The listing builds one solid part. Answer for the finished solid, in the listing's coordinates (mm). A direction names the side the tool comes from. Give positions to 0.01 mm unless a question says otherwise; leave off trailing zeros. Loops run counter-clockwise (first coordinate to the right, second up) from the corner with the lowest first, then second, coordinate; pieces in that order, holes last. Notation, with made-up numbers: M -6,40.25 L 3,40.25 A36 cw 3,77.25 Z; hole C 3,64.25 d5. An arc over 180 degrees is marked long. Return JSON: item names as keys, results as strings.
Autodesk Inventor part; units mm, degrees
ref_plane "YZ Plane" through (0, 0, 0) normal (1, 0, 0) x (0, 1, 0)
ref_plane "XZ Plane" through (0, 0, 0) normal (0, 1, 0) x (-1, 0, 0)
ref_plane "XY Plane" through (0, 0, 0) normal (0, 0, 1) x (1, 0, 0)
sketch "Boceto1" plane through (0, 0, 0) normal (0, 0, 1) x (-1, 0, 0)
  line L0 (-18.5763, -36.3749) -> (-15.5263, -36.3749)
  line L1 (-15.5263, -36.3749) -> (-15.5263, -48.4733)
  line L2 (-15.5263, -48.4733) -> (-5.0037, -48.4733)
  line L3 (-5.0037, -48.4733) -> (-5.0037, -45.4233)
  line L4 (-5.0037, -45.4233) -> (7.1965, -45.4233)
  line L5 (7.1965, -45.4233) -> (7.1965, -48.4733)
  line L6 (7.1965, -48.4733) -> (9.5287, -48.4733)
  line L7 (9.5287, -48.4733) -> (16.194, -48.4733)
  line L8 (16.194, -48.4733) -> (16.194, -47.9303)
  line L9 (16.194, -47.9303) -> (16.194, -45.4233)
  line L10 (16.194, -45.4233) -> (16.194, -36.3411)
  line L11 (16.194, -36.3411) -> (19.2441, -36.3411)
  line L12 (19.2441, -36.3411) -> (19.2441, -24.1748)
  line L13 (19.2444, -24.1748) -> (16.1963, -24.1748)
  line L14 (16.1963, -24.1748) -> (16.1954, -10.116)
  line L15 (16.1954, -10.116) -> (16.194, -6.0779)
  line L16 (16.1918, -6.1454) -> (16.194, -6.0779)
  line L17 (16.194, -6.0779) -> (19.2441, -6.0779)
  line L18 (19.2441, -6.0779) -> (19.2441, 6.1222)
  line L19 (19.2441, 6.1222) -> (16.194, 6.1222)
  line L20 (16.194, 6.1222) -> (16.194, 24.2191)
  line L21 (16.194, 24.2191) -> (19.2441, 24.2191)
  line L22 (19.2441, 24.2191) -> (19.2441, 36.4192)
  line L23 (19.2441, 36.4192) -> (16.194, 36.4192)
  line L24 (16.194, 36.4192) -> (16.194, 45.4676)
  line L25 (16.194, 45.4676) -> (16.194, 48.5176)
  line L26 (16.194, 48.5176) -> (7.1965, 48.5176)
  line L27 (7.1965, 48.5176) -> (7.1965, 45.4676)
  line L28 (7.1965, 45.4676) -> (-3.3262, 45.4676)
  line L29 (-3.3262, 45.4676) -> (-5.0037, 45.4676)
  line L30 (-5.0037, 45.4676) -> (-5.0037, 48.5176)
  line L31 (-5.0037, 48.5176) -> (-15.5263, 48.5176)
  line L32 (-15.5263, 48.5176) -> (-15.5263, 36.4192)
  line L33 (-15.5263, 36.4192) -> (-18.5763, 36.4192)
  line L34 (-18.5763, 36.4192) -> (-18.5763, 24.2191)
  line L35 (-18.5763, 24.2191) -> (-15.5263, 24.2191)
  line L36 (-15.5263, 24.2191) -> (-15.5263, 6.1222)
  line L37 (-15.5263, 6.1222) -> (-18.5763, 6.1222)
  line L38 (-18.5763, 6.1222) -> (-18.5763, -6.0779)
  line L39 (-18.5763, -6.0779) -> (-15.5263, -6.0779)
  line L40 (-15.5263, -6.0779) -> (-15.5263, -24.1748)
  line L41 (-15.5263, -24.1748) -> (-17.5596, -24.1748)
  line L42 (-17.5596, -24.1748) -> (-18.5763, -24.1748)
  line L43 (-18.5763, -24.1748) -> (-18.5763, -36.3749)
  line L44 (-16.0528, -24.1739) -> (-19.1028, -24.1739)
  line L45 (6.6699, 45.4684) -> (4.9416, 45.4684)
  line L46 (-3.8527, -18.4805) -> (-3.8527, -26.614)
  line L47 (-3.8527, -26.614) -> (-6.9027, -26.614)
  line L48 (-6.9027, -26.614) -> (-6.9027, -18.4805)
  line L49 (-6.9027, -18.4805) -> (-3.8527, -18.4805)
  circle A0 centre (1.129, 6.6314) radius 1.0167
  circle A1 centre (4.8907, 0.023) radius 4.575
  circle A2 centre (12.5158, 0.023) radius 1.0167
  circle A3 centre (1.129, -6.5854) radius 1.0167
  point P0 (0, 0)
  dimension "d2" = 96.991
  dimension "d3" = 37.82
extrude "Extrusión1" add sketch "Boceto1" along normal blind 3
properties part number "costat3"
(1) Given pin 1 (1.5 mm diameter, centred on y = 19.5, z = 1.5, fed in from -X); pin 2 (2.5 mm diameter, centred on x = -1.13, y = 6.59, fed in from -Z); pin 3 (0.9 mm diameter, centred on x = -17, z = 1, fed in from +Y), each flat-ended and moving along its own axis, determine where each tip first touches the part or whether it passes through.
Values follow:
{"pin 1": "x = -16.2", "pin 2": "z = 0", "pin 3": "y = 36.34"}
(2) The part is cut by section C-C (z = 1.1). Give the number of separate pieces and of enclosed holes in the cut face, and give its area (3 significant figures).
Values follow:
{"separate pieces": "1", "enclosed holes": "5", "area": "3,130 mm²"}
(3) A tool of negligible diameter and unlimited length cuts with its end or side. For faces 4 (the flat face through (-18, -36.419, 1)), 5 (the flat face through (-16.194, -15, 1)), 6 (the flat face through (-7.196, 47, 1)), 7 (the flat face through (17, 6.078, 1)), from which of +Z, -Z, +X, -X, +Y, -Y can it reach the whole face along a straight path? Write none if from no direction.
Values follow:
{"face 4": "+Z, -Z, -X, -Y", "face 5": "+Z, -Z, -X", "face 6": "+Z, -Z, +Y", "face 7": "+Z, -Z, +X"}
(4) The part is cut by section B-B (y = 38). Determine the outline of the cut face in (x, z), and give its area (3 significant figures).
Values follow:
{"outline": "M -16.19,0 L 15.53,0 L 15.53,3 L -16.19,3 Z", "area": "95.2 mm²"}
(5) The part is cut by section A-A (y = 2). Determine the outline of the cut face in (x, z).
Values follow:
{"outline": "M -19.24,0 L -8.99,0 L -8.99,3 L -19.24,3 Z; M -0.79,0 L 18.58,0 L 18.58,3 L -0.79,3 Z"}
(6) Straight lines are drawn through the part: line 1 along X through (y, z) = (0, 0.5); line 2 along Y through (x, z) = (-18, 0.4); line 3 along Y through (x, z) = (-1, 1.7). For each, find the intervals that lie inside material, in ascending order.
Values follow:
{"line 1": "-19.24 to -13.53, -11.5 to -9.47, -0.32 to 18.58", "line 2": "-36.42 to -24.22, -6.12 to 6.08, 24.17 to 36.34", "line 3": "-45.47 to -7.64, -5.62 to -2.43, 2.38 to 5.58, 7.59 to 45.42"}
(7) Determine the mould class of faces 1 (the flat face through (17, 36.375, 1)), 2 (the flat face through (18.576, 0, 1)), 3 (the flat face through (5.004, -47, 1)) for opening direction X: released by +X, released by -X, zero draft, split by the parting line, or undercut.
Values follow:
{"face 1": "zero draft", "face 2": "released by +X", "face 3": "undercut"}
(8) The part is cut by section D-D (y = 14.5). Determine the outline of the cut face in (x, z).
Values follow:
{"outline": "M -16.2,0 L 15.53,0 L 15.53,3 L -16.2,3 Z"}
